```python
from build123d import *

# Parameters (mm, degrees)
SKETCH1_R           = 187.5
BOSS_EXTRUDE1_DEPTH = 282
SKETCH2_W           = 150
SKETCH2_H           = 210
BOSS_EXTRUDE2_DEPTH = 10
SKETCH3_W           = 150
SKETCH3_H           = 210
BOSS_EXTRUDE3_DEPTH = 10
BOSS_EXTRUDE4_REACH = 294
SKETCH4_W           = 150
SKETCH4_H           = 10
SKETCH5_R           = 75
BOSS_EXTRUDE5_DEPTH = 152.4
SKETCH8_R           = 3.8
SKETCH9_R           = 3.8
BOSS_EXTRUDE6_DEPTH = 283.8


with BuildPart() as part:
    # Sketch1 → Boss-Extrude1 (new body)
    with BuildSketch(Plane(origin=(0, 0, 0), x_dir=(0, 0, -1), z_dir=(1, 0, 0))):
        Circle(SKETCH1_R)
    extrude(amount=BOSS_EXTRUDE1_DEPTH)

    # Sketch2 → Boss-Extrude2 (add)
    with BuildSketch(Plane.ZY):
        with Locations((0, -105)):
            Rectangle(SKETCH2_W, SKETCH2_H)
    extrude(amount=BOSS_EXTRUDE2_DEPTH)

    # Sketch3 → Boss-Extrude3 (add)
    with BuildSketch(Plane(origin=(282, 0, 0), x_dir=(0, 0, -1), z_dir=(1, 0, 0))):
        with Locations((0, -105)):
            Rectangle(SKETCH3_W, SKETCH3_H)
    extrude(amount=BOSS_EXTRUDE3_DEPTH)

    # Sketch4 → Boss-Extrude4 (add, up to next)
    with BuildSketch(Plane(origin=(0, 0, 0), x_dir=(0, 0, -1), z_dir=(1, 0, 0)), mode=Mode.PRIVATE) as boss_extrude4_sk1:
        with Locations((0, -205)):
            Rectangle(SKETCH4_W, SKETCH4_H)
    boss_extrude4_tool1 = extrude(boss_extrude4_sk1.sketch, amount=BOSS_EXTRUDE4_REACH, mode=Mode.PRIVATE) - part.part
    add(boss_extrude4_tool1.solids().sort_by_distance((0, -205, 0))[0])

    # Sketch5 → Boss-Extrude5 (add)
    with BuildSketch(Plane.ZY.offset(10)):
        Circle(SKETCH5_R)
    extrude(amount=BOSS_EXTRUDE5_DEPTH)

    # Sweep2: sweep along a path in Sketch6
    with BuildLine(Plane(origin=(50.7, 0, 0), x_dir=(0, 0, -1), z_dir=(1, 0, 0))) as sweep2_path:
        Line((0, -187.5), (-200, -187.5))
    # Sketch8 → Sweep2 (sweep)
    with BuildSketch(Plane.XY.offset(200)):
        with Locations((50.7, -187.5)):
            Circle(SKETCH8_R)
    sweep(path=sweep2_path.line)

    # Sketch9 → Boss-Extrude6 (add)
    with BuildSketch(Plane.XY.offset(200)):
        with Locations((50.7, -187.5)):
            Circle(SKETCH9_R)
    extrude(amount=BOSS_EXTRUDE6_DEPTH)


solid = part.part
```
Verification items for the finished model (mm, model axes). A direction names the side the tool comes from. Give positions to 0.01 mm unless a question says otherwise; leave off trailing zeros. Loops run counter-clockwise (first coordinate to the right, second up) from the corner with the lowest first, then second, coordinate; pieces in that order, holes last.
1. Go/stop test with flat-tipped pins: pin 1 Ø8 at (x, z) = (289, -20.5) entering from +Y; pin 2 Ø1 at (y, z) = (-35.5, 84) entering from +X; pin 3 Ø6 at (x, y) = (-23.5, -31) entering from -Z. Record where each tip stops, or that it passes through.
2. Mould release check, pull along Y, two halves, no side actions. Record for faces 6 (the flat face through (139, -210, 1)), 7 (the flat face through (-162.4, 1, -1)), 8 (the flat face through (0, -192, -1)): released by +Y, released by -Y, zero draft, split by the parting line, or undercut.
3. Section check C-C, the plane x = 182.5. Enter the section's corners in (y, z).
4. Section check A-A, the plane y = 66. Enter the section's corners in (x, z).
5. Set-up check for faces 1 (the flat face through (-10, 30, -1)), 2 (the flat face through (140, -207, 75)), 3 (the flat face through (282, -192, 1)), 4 (the flat face through (140, -207, -75)), 5 (the flat face through (139, -200, 1)): record each of +Z, -Z, +X, -X, +Y, -Y from which the full face is reachable in a straight line by a thin tool's end or side.
6. Section check B-B, the plane z = 32.5. Enter the section's corners in (x, y), then the cut area to 3 significant figures.
7. Thickness scan on line 1 (X direction, y = -188.5, z = 61.5); line 2 (X direction, y = -193, z = 65); line 3 (Z direction, x = -9.5, y = -122.5). Record the ranges inside material, lowest first.
8. Section check D-D, the plane z = 293. Enter the section's corners in (x, y), then the cut area to 3 significant figures.
Geometry says:
1. pin 1: stops at y = 0
1. pin 2: stops at x = 282
1. pin 3: stops at z = -69.58
2. face 6: released by -Y
2. face 7: zero draft
2. face 8: undercut
3. outline: (-210, -75) - (-200, -75) - (-200, 75) - (-210, 75) - close; circle Ø375 at (0, 0)
4. outline: (-162.4, -35.62) - (-10, -35.62) - (-10, 35.62) - (-162.4, 35.62) - close; (0, -175.5) - (282, -175.5) - (282, 175.5) - (0, 175.5) - close
5. face 1: +Z, -Z, +Y
5. face 2: +Z, -Y
5. face 3: none
5. face 4: -Z, -Y
5. face 5: +Z, -Z
6. outline: (-162.4, -67.59) - (-10, -67.59) - (-10, -210) - (292, -210) - (292, 0) - (282, 0) - (282, 184.66) - (0, 184.66) - (0, 0) - (-10, 0) - (-10, 67.59) - (-162.4, 67.59) - close; hole (0, -200) - (282, -200) - (282, -184.66) - (53.23, -184.66) arc R3.8 cw (long way) to (48.17, -184.66) - (0, -184.66) - close
6. area: 132,000 mm2
7. line 1: x = -10 to 0, 47.03 to 54.37, 282 to 292
7. line 2: x = -10 to 0, 282 to 292
7. line 3: z = -75 to 75
8. outline: circle Ø7.6 at (50.7, -187.5)
8. area: 45.4 mm2
